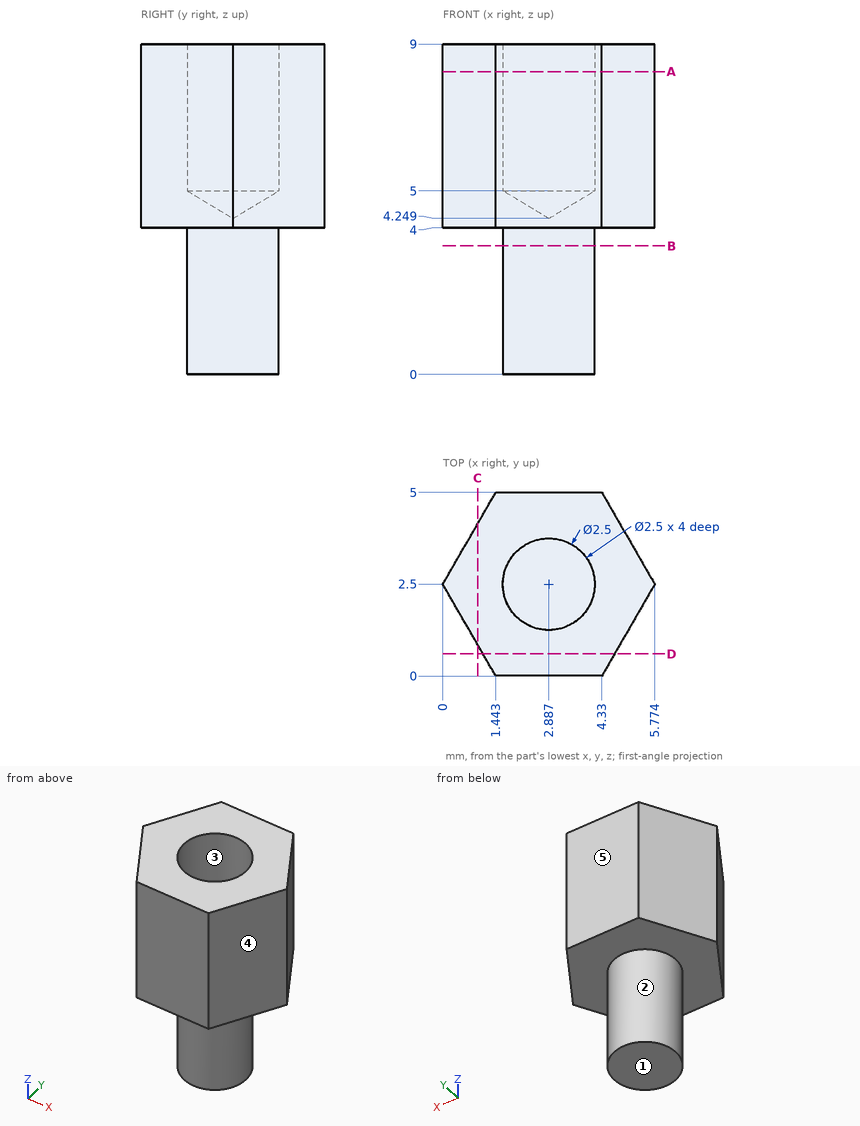
Here's the drawing with two shaded views (mm, measured from the low corner). I have some questions. A direction names the side the tool comes from. Give positions to 0.01 mm unless a question says otherwise; leave off trailing zeros. Write each loop counter-clockwise with the first axis right and the second up, starting at its lowest first coordinate (ties: lowest second). Pieces come first, ordered by that corner, then holes. Notation, with made-up numbers: (-16, 59.25) -> (7, 59.25) arc R28 cw to (7, 82.25) -> close; hole circle Ø8 at (-15, 12.5). An arc over 180 degrees is marked (long way). Answer as a JSON object with one key per item and string values. Group by question number.
Item 1: For the marked faces 1 and 2, which set-ups out of +Z, -Z, +X, -X, +Y, -Y let a thin tool reach every point of the face, with its end or its side?
Item 2: I'm going to push flat-ended pins straight in: P1, Ø1, axis at x = 5, y = 1, coming from the -Z side; P2, Ø1.5, axis at y = 1.5, z = 3, coming from the -X side; P3, Ø2.5, axis at x = 3, y = 3, coming from the -Z side. Where does each tip first touch, or does it pass through?
Item 3: Suppose I cut it at D-D (y = 0.6). Please give me the cut outline in (x, z), plus the area to 3 significant figures.
Item 4: Suppose I cut it at A-A (z = 8.25). Please give me the cut outline in (x, y).
Item 5: Please list where these lines run through material, in increasing order: line 1 (Y direction, x = 2.9, z = 7.5); line 2 (Z direction, x = 3.9, y = 3.6); line 3 (X direction, y = 2.3, z = 6) (1 decimal). Write a range as [from, to].
Item 6: Suppose I cut it at C-C (x = 0.95). Please give me the cut outline in (y, z) (1 decimal).
Item 7: Suppose I cut it at B-B (z = 3.5). Please give me the cut outline in (x, y).
Item 8: We'd pull the mould along X, two halves only. Please class the marked faces 3, 4 and 5: +X half, -X half, draft (parallel to the pull), parting line (faces both ways), or undercut.
Findings:
{
 "1": {"face 1": "-Z, +X, -X, +Y, -Y", "face 2": "-Z"},
 "2": {"P1": "stops at z = 4", "P2": "stops at x = 1.66", "P3": "stops at z = 0"},
 "3": {"outline": "(1.1, 4) -> (4.68, 4) -> (4.68, 9) -> (1.1, 9) -> close", "area": "17.9 mm²"},
 "4": {"outline": "(0, 2.5) -> (1.44, 0) -> (4.33, 0) -> (5.77, 2.5) -> (4.33, 5) -> (1.44, 5) -> close; hole circle Ø2.5 at (2.89, 2.5)"},
 "5": {"line 1": "y = [0, 1.25], [3.75, 5]", "line 2": "z = [4, 9]", "line 3": "x = [0.1, 1.7], [4.1, 5.7]"},
 "6": {"outline": "(0.9, 4) -> (4.1, 4) -> (4.1, 9) -> (0.9, 9) -> close"},
 "7": {"outline": "circle Ø2.5 at (2.89, 2.5)"},
 "8": {"face 3": "undercut", "face 4": "+X half", "face 5": "draft"}
}
